Autodesk Inventor part; units mm, degrees
ref_plane "YZ Plane" through (0, 0, 0) normal (1, 0, 0) x (0, 1, 0)
ref_plane "XZ Plane" through (0, 0, 0) normal (0, 1, 0) x (-1, 0, 0)
ref_plane "XY Plane" through (0, 0, 0) normal (0, 0, 1) x (1, 0, 0)
sketch "Sketch1" plane through (0, 0, 0) normal (0, 1, 0) x (-1, 0, 0)
  line L0 (0, 0) -> (12.6, 0)
  line L1 (12.6, 0) -> (12.6, 22.3)
  line L2 (0, 0) -> (0, 22.3)
  line L3 (0, 22.3) -> (3.9, 35)
  line L4 (3.9, 35) -> (8.7, 35)
  line L5 (8.7, 35) -> (12.6, 22.3)
  point P0 (6.3, 6.5)
  dimension "d4" = 22.3
  dimension "d5" = 4.8
extrude "Extrusion1" add sketch "Sketch1" along normal blind 4.8
sketch "Sketch2" plane through (0, 0, 0) normal (0, -1, 0) x (1, 0, 0)
  point P0 (0, 0)
  point P1 (-6.3, 6.5)
hole "Hole1" at (-6.3, 0, 6.5) direction (0, 1, 0) diameter 4.2 depth 8 tip angle 118 countersink diameter 8.4 countersink angle 90
sketch "Sketch3" plane through (0, 0, 0) normal (0, -1, 0) x (1, 0, 0)
  circle A0 centre (-6.3, 19.5) radius 2.3
  point P0 (0, 0)
  dimension "d13" = 4.6
extrude "Extrusion2" cut sketch "Sketch3" against normal through all
sketch "Sketch4" plane through (0, 0, 0) normal (1, 0, 0) x (0, 1, 0)
  line L0 (0, 35) -> (4.8, 35)
  line L1 (0, 22.3) -> (4.8, 22.3)
  line L2 (4.8, 22.3) -> (2.4, 35)
  line L3 (4.8, 35) -> (4.8, 22.3)
  line L4 (2.4, 35) -> (4.8, 35)
  line L5 (4.8, 35) -> (4.8, 22.3)
  point P0 (0, 0)
extrude "Extrusion3" cut sketch "Sketch4" against normal through all
sketch "Sketch5" plane through (0, 0, 0) normal (1, 0, 0) x (0, 1, 0)
  point P0 (0, 0)
sketch "Sketch6" plane through (0, 0, 0) normal (0, -1, 0) x (1, 0, 0)
  line L0 (-8.7, 35) -> (-3.9, 35)
  line L1 (-4.9584, 35) -> (-7.4584, 35)
  line L2 (-7.4584, 35) -> (-7.4584, 33)
  line L3 (-7.4584, 33) -> (-4.9584, 33)
  line L4 (-4.9584, 33) -> (-4.9584, 35)
  point P0 (0, 0)
  point P1 (-6.3, 35)
  dimension "d18" = 2.5
  dimension "d19" = 2
extrude "Extrusion4" cut sketch "Sketch6" against normal blind 1.27
properties part number "HeadbarClampBottom"
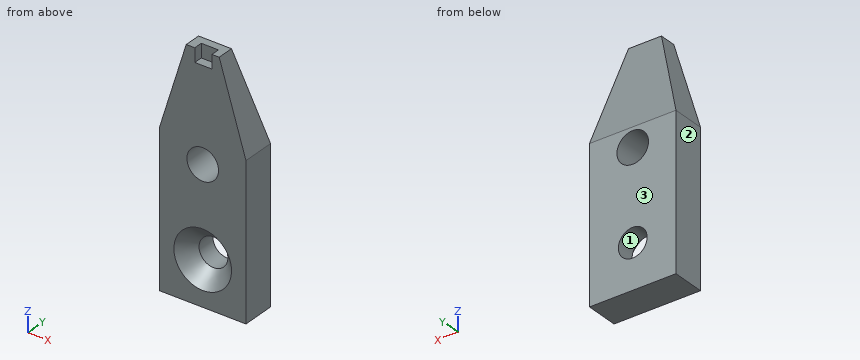
Can you work these out from the model? Positions are in its coordinate system, mm. Face numbers are marked on the shaded views. Coordinates: 2 decimals unless noted, no trailing zeros. Loops run counter-clockwise (first coordinate to the right, second up) from the corner with the lowest first, then second, coordinate; pieces in that order, holes last.
1) Thinking about a two-plate mould opening in X: for the marked faces 1, 2 and 3, which applies, pulls with the +X half, pulls with the -X half, needs draft (parallel to the pull), parting line crosses it, or undercut?
2) Imagine slicing it at D-D on y = 3.9. List the corners of the cut face in (x, z) for me, plus the area to 3 significant figures.
3) Imagine slicing it at C-C on z = 19.5. List the corners of the cut face in (x, y) for me.
4) For pin 1 (1.4 mm diameter, centred on y = 0.5, z = 34.5, fed in from -X); pin 2 (1.4 mm diameter, centred on y = 0.5, z = 34.5, fed in from +X); pin 3 (1.5 mm diameter, centred on x = -11.5, z = 23.5, fed in from +Y), each with a flat end and sliding along its axis, tell me the tip position at first contact or that it passes through.
5) Imagine slicing it at A-A on z = 6.5. List the corners of the cut face in (x, y) for me.
6) I need wall thicknesses on probe 1 along X at (y, z) = (4, 6.5); probe 2 along Z at (x, y) = (-7.25, 1.65); probe 3 along X at (y, z) = (1.15, 20) (3 decimals). Which ranges of each line are inside material? Lowest first, please.
7) Imagine slicing it at B-B on x = -6.3. List the corners of the cut face in (y, z) for me, plus the area to 3 significant figures.
Completed:
1. face 1: undercut
1. face 2: pulls with the -X half
1. face 3: needs draft
2. outline: (-12.6, 0) - (0, 0) - (0, 22.3) - (-1.46, 27.06) - (-11.14, 27.06) - (-12.6, 22.3) - close; hole circle Ø4.6 at (-6.3, 19.5); hole circle Ø4.2 at (-6.3, 6.5)
2. area: 304 mm2
3. outline: (-12.6, 0) - (-8.6, 0) - (-8.6, 4.8) - (-12.6, 4.8) - close; (-4, 0) - (0, 0) - (0, 4.8) - (-4, 4.8) - close
4. pin 1: stops at x = -9.07
4. pin 2: stops at x = -3.53
4. pin 3: stops at y = 4.71
5. outline: (-12.6, 0) - (-10.5, 0) - (-8.4, 2.1) - (-8.4, 4.8) - (-12.6, 4.8) - close; (-4.2, 2.1) - (-2.1, 0) - (0, 0) - (0, 4.8) - (-4.2, 4.8) - close
6. probe 1: x = -12.6 to -8.4, -4.2 to 0
6. probe 2: z = 0 to 4.13, 8.87 to 17.41, 21.59 to 35
6. probe 3: x = -12.6 to -8.545, -4.055 to 0
7. outline: (0, 0) - (4.8, 0) - (4.8, 4.4) - (2.1, 4.4) - (0, 2.3) - close; (0, 10.7) - (2.1, 8.6) - (4.8, 8.6) - (4.8, 17.2) - (0, 17.2) - close; (0, 21.8) - (4.8, 21.8) - (4.8, 22.3) - (2.4, 35) - (1.27, 35) - (1.27, 33) - (0, 33) - close
7. area: 104 mm2
